The model under review builds one solid part; all positions refer to its coordinate system, in mm. A direction names the side the tool comes from. Give positions to 0.01 mm unless a question says otherwise; leave off trailing zeros. Loops run counter-clockwise (first coordinate to the right, second up) from the corner with the lowest first, then second, coordinate; pieces in that order, holes last. Notation, with made-up numbers: M 26,15 L 33,15 A15 ccw 33,34 Z; hole C 53.25,-23 d1. An arc over 180 degrees is marked long. Return JSON: item names as keys, results as strings. Group by question number.
```python
from build123d import *

# Parameters (mm, degrees)
SKETCH1_W           = 600
SKETCH1_H           = 400
BOSS_EXTRUDE1_DEPTH = 200
CUT_EXTRUDE1_DEPTH  = 190
SKETCH3_R           = 11
CUT_EXTRUDE2_DEPTH  = 10
SKETCH4_R           = 12
SKETCH4_R_2         = 8
CUT_EXTRUDE3_DEPTH  = 10
SKETCH5_W           = 47
SKETCH5_H           = 27
CUT_EXTRUDE4_DEPTH  = 10
SKETCH6_R           = 11
CUT_EXTRUDE5_DEPTH  = 10


with BuildPart() as part:
    # Sketch1 → Boss-Extrude1 (new body)
    with BuildSketch(Plane(origin=(0, 0, 0), x_dir=(1, 0, 0), z_dir=(0, 1, 0))):
        Rectangle(SKETCH1_W, SKETCH1_H)
    extrude(amount=BOSS_EXTRUDE1_DEPTH)

    # Sketch2 → Cut-Extrude1 (cut)
    with BuildSketch(Plane(origin=(0, 200, 0), x_dir=(1, 0, 0), z_dir=(0, 1, 0))):
        Polygon((-224, -197), (224, -197), (224, -176), (276, -176), (276, -138), (297, -138), (297, 138), (276, 138), (276, 176), (224, 176), (224, 197), (-224, 197), (-224, 176), (-276, 176), (-276, 138), (-297, 138), (-297, -138), (-276, -138), (-276, -176), (-224, -176), align=None)
    extrude(amount=-CUT_EXTRUDE1_DEPTH, mode=Mode.SUBTRACT)

    # Sketch3 → Cut-Extrude2 (cut)
    with BuildSketch(Plane.ZY.offset(300)):
        with Locations((-100, 100)):
            Circle(SKETCH3_R)
        with Locations((-50, 100)):
            Circle(SKETCH3_R)
        with Locations((50, 100)):
            Circle(SKETCH3_R)
        with Locations((100, 100)):
            Circle(SKETCH3_R)
        with Locations((0, 100)):
            Circle(SKETCH3_R)
    extrude(amount=-CUT_EXTRUDE2_DEPTH, mode=Mode.SUBTRACT)

    # Sketch4 → Cut-Extrude3 (cut)
    with BuildSketch(Plane.XY.offset(200)):
        with Locations((150, 100)):
            Circle(SKETCH4_R)
        with Locations((75, 100)):
            Circle(SKETCH4_R_2)
        with Locations((225, 100)):
            Circle(SKETCH4_R)
        with Locations((0, 100)):
            Circle(SKETCH4_R_2)
        with Locations((190, 100)):
            Circle(SKETCH4_R)
    extrude(amount=-CUT_EXTRUDE3_DEPTH, mode=Mode.SUBTRACT)

    # Sketch5 → Cut-Extrude4 (cut)
    with BuildSketch(Plane(origin=(0, 0, -200), x_dir=(-1, 0, 0), z_dir=(0, 0, -1))):
        with Locations((-225, 100)):
            Rectangle(SKETCH5_W, SKETCH5_H)
    extrude(amount=-CUT_EXTRUDE4_DEPTH, mode=Mode.SUBTRACT)

    # Sketch6 → Cut-Extrude5 (cut)
    with BuildSketch(Plane(origin=(300, 0, 0), x_dir=(0, 0, -1), z_dir=(1, 0, 0))):
        with Locations((0, 133)):
            Circle(SKETCH6_R)
    extrude(amount=-CUT_EXTRUDE5_DEPTH, mode=Mode.SUBTRACT)


solid = part.part
```
(1) Add section B-B (y = 23.5). Write out the cut boundary in (x, z), and give its area (3 significant figures).
(2) For probe 1 along Z at (x, y) = (79, 117.5); probe 2 along X at (y, z) = (92, 140); probe 3 along X at (y, z) = (48.5, 131), list the stretches that pass through material, from the lowest coordinate up.
(3) Add section D-D (z = 0). Write out the cut boundary in (x, y).
(4) For faces 1 (the cylindrical face through (-299, 100, -111)), 2 (the flat face through (3, 106, -197)), 3 (the cylindrical face through (298.521, 143.906, 1.432)), 4 (the flat face through (-4, 99, -200)), 5 (the cylindrical face through (-1.73, 92.19, 198.52)), list the 3-axis set-ups (+Z, -Z, +X, -X, +Y, -Y) from which the entire face can be reached by the end or side of a thin tool; tool diameter is ignored.
(5) Mouldability with a two-part tool opening along Y and no side actions: class faces 6 (the flat face through (-250, 106, -176)), 7 (the cylindrical face through (68.651, 95.132, 198.521)), 8 (the flat face through (-4, 0, -3)) as released by +Y, released by -Y, zero draft, split by the parting line, or undercut.
(6) Add section C-C (x = 0). Write out the cut boundary in (y, z), and give its area (3 significant figures).
(7) Add section A-A (z = 100). Write out the cut boundary in (x, y).
(8) For pin 1 (17.5 mm diameter, centred on y = 100, z = -100, fed in from -X); pin 2 (19 mm diameter, centred on x = 150, y = 100, fed in from +Z); pin 3 (2 mm diameter, centred on x = 229, z = 14, fed in from +Y), all flat-tipped, find the tip position at first contact; note any pin that passes through.
Verdict:
{
 "1": {"outline": "M -300,-200 L 300,-200 L 300,200 L -300,200 Z; hole M -297,-138 L -276,-138 L -276,-176 L -224,-176 L -224,-197 L 224,-197 L 224,-176 L 276,-176 L 276,-138 L 297,-138 L 297,138 L 276,138 L 276,176 L 224,176 L 224,197 L -224,197 L -224,176 L -276,176 L -276,138 L -297,138 Z", "area": "15,300 mm²"},
 "2": {"probe 1": "z = -200 to -197, 197 to 200", "probe 2": "x = -300 to -276, 276 to 300", "probe 3": "x = -300 to -297, 297 to 300"},
 "3": {"outline": "M -300,0 L 300,0 L 300,122 L 297,122 L 297,10 L -297,10 L -297,89 L -300,89 Z; M -300,111 L -297,111 L -297,200 L -300,200 Z; M 297,144 L 300,144 L 300,200 L 297,200 Z"},
 "4": {"face 1": "-X", "face 2": "+Y", "face 3": "+X", "face 4": "-Z, +X, -X, +Y, -Y", "face 5": "+Z"},
 "5": {"face 6": "zero draft", "face 7": "undercut", "face 8": "released by -Y"},
 "6": {"outline": "M 0,-200 L 200,-200 L 200,-197 L 10,-197 L 10,197 L 92,197 L 92,200 L 0,200 Z; M 108,197 L 200,197 L 200,200 L 108,200 Z", "area": "5,090 mm²"},
 "7": {"outline": "M -300,0 L 300,0 L 300,200 L 297,200 L 297,10 L -297,10 L -297,89 L -300,89 Z; M -300,111 L -297,111 L -297,200 L -300,200 Z"},
 "8": {"pin 1": "stops at x = 297", "pin 2": "stops at z = -197", "pin 3": "stops at y = 10"}
}
